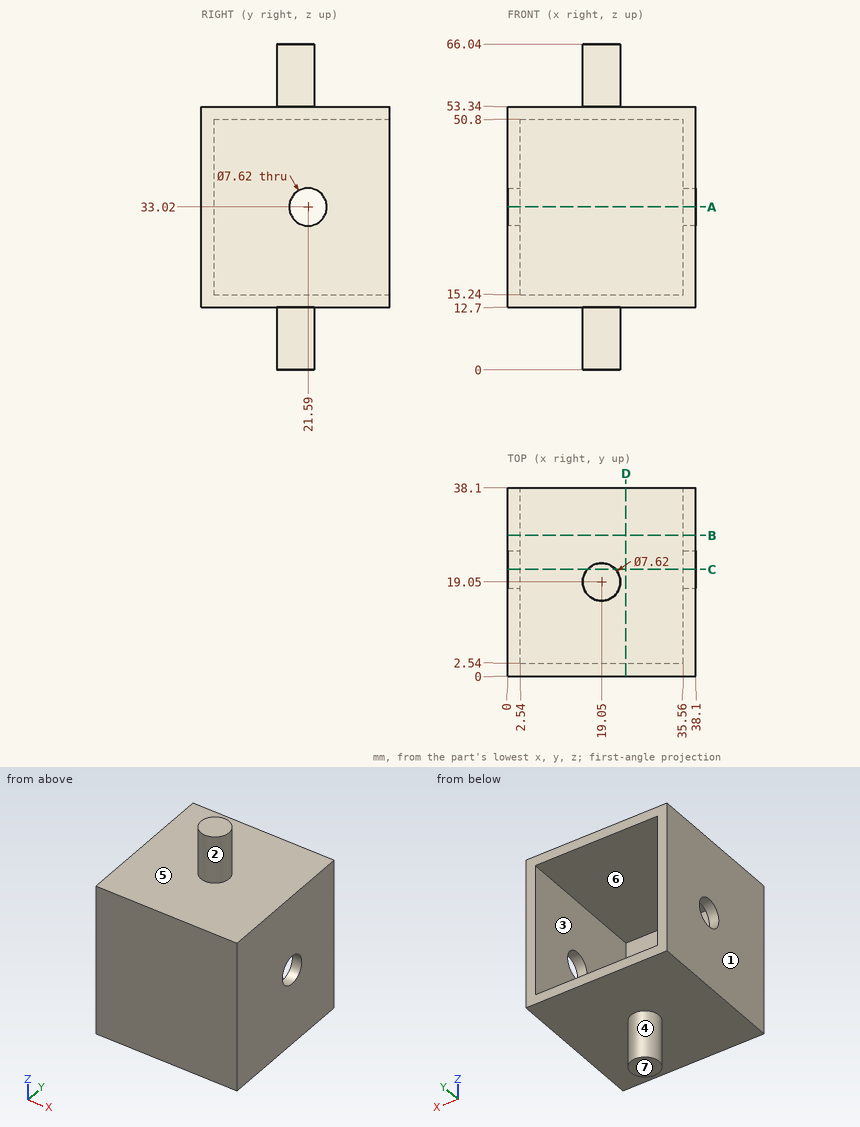
Could you check a few things on this drawing? It's one solid part, dimensions in mm from its lowest x, y, z. A direction names the side the tool comes from. Coordinates: 2 decimals unless noted, no trailing zeros. Order: outer loops, then holes, each group sorted by start corner. A loop starts at its lowest first (then second) coordinate and runs counter-clockwise, first axis right, second up. Notation, with made-up numbers: M 54.25,78.5 L 63.25,78.5 A33 cw 63.25,113.5 Z; hole C 58.25,22.5 d4. An arc over 180 degrees is marked long. Use one line per item in the form item = value. Start each with the question number.
1. For pin 1 (10 mm diameter, centred on x = 34, y = 33, fed in from -Z); pin 2 (10 mm diameter, centred on x = 6.5, y = 7, fed in from +Z); pin 3 (6 mm diameter, centred on y = 21.59, z = 33.02, fed in from +X); pin 4 (16.5 mm diameter, centred on x = 12.5, z = 33, fed in from +Y), each with a flat end and sliding along its axis, tell me the tip position at first contact or that it passes through.
2. Suppose I cut it at B-B on y = 28.5. Write out the boundary of the cut face in (x, z).
3. On a 3-axis mill with a long thin cutter (end or side, diameter ignored), from which of +Z, -Z, +X, -X, +Y, -Y can I reach the whole of each face in a straight line? I mean the marked faces 1, 2, 3 and 4. Say none if no direction works.
4. Suppose I cut it at C-C on y = 21.59. Write out the boundary of the cut face in (x, z).
5. Suppose I cut it at A-A on z = 33.02. Write out the boundary of the cut face in (x, y).
6. We'd pull the mould along Z, two halves only. Please class the marked faces 5, 6 and 7: +Z half, -Z half, draft (parallel to the pull), parting line (faces both ways), or undercut.
7. Suppose I cut it at D-D on x = 24. Write out the boundary of the cut face in (y, z).
8. Please list where these lines run through material, in increasing order: line 1 (X direction, y = 14, z = 19.5); line 2 (Y direction, x = 1, z = 33); line 3 (Z direction, x = 22.5, y = 16).
Geometry says:
q1.pin_1 = 12.7
q1.pin_2 = 53.34
q1.pin_3 = through
q1.pin_4 = 2.54
q2.outline = M 0,12.7 L 38.1,12.7 L 38.1,53.34 L 0,53.34 Z; hole M 2.54,15.24 L 35.56,15.24 L 35.56,50.8 L 2.54,50.8 Z
q3.face_1 = +Z, -Z, -X, +Y, -Y
q3.face_2 = +Z
q3.face_3 = +Y
q3.face_4 = -Z
q4.outline = M 0,12.7 L 16.21,12.7 L 16.21,0 L 21.89,0 L 21.89,12.7 L 38.1,12.7 L 38.1,29.21 L 35.56,29.21 L 35.56,15.24 L 2.54,15.24 L 2.54,29.21 L 0,29.21 Z; M 0,36.83 L 2.54,36.83 L 2.54,50.8 L 35.56,50.8 L 35.56,36.83 L 38.1,36.83 L 38.1,53.34 L 21.89,53.34 L 21.89,66.04 L 16.21,66.04 L 16.21,53.34 L 0,53.34 Z
q5.outline = M 0,0 L 38.1,0 L 38.1,17.78 L 35.56,17.78 L 35.56,2.54 L 2.54,2.54 L 2.54,17.78 L 0,17.78 Z; M 0,25.4 L 2.54,25.4 L 2.54,38.1 L 0,38.1 Z; M 35.56,25.4 L 38.1,25.4 L 38.1,38.1 L 35.56,38.1 Z
q6.face_5 = +Z half
q6.face_6 = undercut
q6.face_7 = -Z half
q7.outline = M 0,12.7 L 38.1,12.7 L 38.1,15.24 L 2.54,15.24 L 2.54,50.8 L 38.1,50.8 L 38.1,53.34 L 0,53.34 Z
q8.line_1 = 0 to 2.54, 35.56 to 38.1
q8.line_2 = 0 to 17.78, 25.4 to 38.1
q8.line_3 = 12.7 to 15.24, 50.8 to 53.34
